Can you work these out from the model? Positions are in its coordinate system, mm. Coordinates: 2 decimals unless noted, no trailing zeros. Loops run counter-clockwise (first coordinate to the right, second up) from the corner with the lowest first, then second, coordinate; pieces in that order, holes last. Notation, with made-up numbers: M 66,-21.5 L 93,-21.5 A20 cw 93,-14.5 Z; hole C 68.5,-22.5 d4. An arc over 180 degrees is marked long. Return JSON: item names as keys, results as strings. Group by question number.
Autodesk Fusion 360 part; units mm, degrees
sketch "Sketch1" plane through (0, 0, 0) normal (0, 0, 1) x (1, 0, 0)
  circle A0 centre (0, 0) radius 7.5
  circle A1 centre (0, 0) radius 9.7
  circle A2 centre (12.825, 0) radius 3.125
  circle A3 centre (12.825, 0) radius 5.325
  line L0 (-19.1275, 0) -> (19.1275, 0) construction
  line L1 (0, 53.4087) -> (0, -53.4087) construction
  circle A4 centre (9.8375, -2.9875) radius 1.1
  circle A5 centre (15.8125, -2.9875) radius 1.1
  circle A6 centre (7.4478, 4.3) radius 1.1
  line L2 (0, 0) -> (7.4478, 4.3) construction
  line L3 (0, 0) -> (12.825, 0) construction
  line L4 (9.8375, -2.9875) -> (12.825, 0) construction
  line L5 (15.8125, -2.9875) -> (12.825, 0) construction
  line L6 (9.8375, -2.9875) -> (15.8125, -2.9875) construction
  dimension "d5_1_1_2_1" = 15
  dimension "d6_1_1_2_1" = 2.2
  dimension "d7_1_1_2_1" = 6.25
  dimension "d9_1_1_2_1" = 2.2
  dimension "d17_1_1_2_1" = 2.2
  dimension "d18_1_1_2_1" = 2.2
  dimension "d23_1_1_2_1" = 2.2
  dimension "d32_1" = 90
  dimension "d34_1" = 90
  dimension "d36" = 30
extrude "Extrude1" add sketch "Sketch1" along normal blind 5 contours A0 A1 A3 A6 | A1 A3 A4 | A6 | A1 A2 A3 A5 | A1 A3 A4 | A1 A2 A4 | A1 A4 | A1 A4 | A5 picked at (6.1847, 5.9307)
fillet "Fillet1" radius 0.5 1 edges at (8.9752, -3.679, 2.5)
chamfer "Chamfer2" distance 0.6 angle 45 16 edges at (10.7426, -3.6127, 5) (9.0094, -3.9762, 5) (-9.6936, -0.3518, 5) (7.9978, 3.3474, 5) (-7.2444, -1.9411, 5) (14.8628, 4.9197, 5) (15.0347, -3.7653, 5) (12.825, 3.125, 5) (10.7426, -3.6127, 0) (9.0094, -3.9762, 0) (-9.6936, -0.3518, 0) (7.9978, 3.3474, 0) (-7.2444, -1.9411, 0) (14.8628, 4.9197, 0) (15.0347, -3.7653, 0) (12.825, 3.125, 0)
equation "d6_1_1_2_1 = ClipWall"
equation "d9_1_1_2_1 = ClipWall"
equation "d17_1_1_2_1 = ClipWall"
equation "d18_1_1_2_1 = ClipWall"
equation "d21_1_1_2_1 = Thickness"
equation "d23_1_1_2_1 = ClipWall"
equation "ClipWall = 2.2 mm"
equation "Thickness = 5 mm"
1) Suppose I cut it at C-C, the plane y = 2.5. Give the number of separate pieces and of enclosed holes in the cut face, then the cut area to 3 significant figures.
2) If we mould it in two halves opening along X, with no side actions, what happens to faces 1 (the face through (10.755, -3.595, 2.473)), 2 (the face through (8.1, -2, 5))? For each: +X half, -X half, draft (parallel to the pull), parting line (faces both ways), or undercut.
3) For pin 1 (9 mm diameter, centred on x = 0, y = 0, fed in from +Z); pin 2 (1 mm diameter, centred on y = -3, z = 3, fed in from -X), each with a flat end and sliding along its axis, tell me the tip position at first contact or that it passes through.
4) If I drill on line 1 (X direction, y = 0, z = 2.4); line 2 (Y direction, x = 0, z = 1.8); line 3 (X direction, y = -5.75, z = 0.85), over which ranges is the centre line in solid material (lowest first)? Write a range as from..to.
5) Suppose I cut it at B-B, the plane y = 0. List the corners of the cut face in (x, z) for me.
6) Suppose I cut it at A-A, the plane x = 0. List the corners of the cut face in (y, z) for me, then the cut area to 3 significant figures.
Returned:
{
 "1": {"separate pieces": "3", "enclosed holes": "0", "area": "37.1 mm²"},
 "2": {"face 1": "undercut", "face 2": "draft"},
 "3": {"pin 1": "passes through", "pin 2": "stops at x = -9.37"},
 "4": {"line 1": "x = -9.7..-7.5, 7.5..9.7, 15.95..18.15", "line 2": "y = -9.7..-7.5, 7.5..9.7", "line 3": "x = -7.81..-4.82, 4.82..7.81"},
 "5": {"outline": "M -9.7,0.6 L -9.1,0 L -8.1,0 L -7.5,0.6 L -7.5,4.4 L -8.1,5 L -9.1,5 L -9.7,4.4 Z; M 7.5,0.6 L 8.1,0 L 9.1,0 L 9.7,0.6 L 9.7,4.4 L 9.1,5 L 8.1,5 L 7.5,4.4 Z; M 15.95,0.6 L 16.55,0 L 17.55,0 L 18.15,0.6 L 18.15,4.4 L 17.55,5 L 16.55,5 L 15.95,4.4 Z"},
 "6": {"outline": "M -9.7,0.6 L -9.1,0 L -8.1,0 L -7.5,0.6 L -7.5,4.4 L -8.1,5 L -9.1,5 L -9.7,4.4 Z; M 7.5,0.6 L 8.1,0 L 9.1,0 L 9.7,0.6 L 9.7,4.4 L 9.1,5 L 8.1,5 L 7.5,4.4 Z", "area": "20.6 mm²"}
}
